Here's how the part is built. I have some questions about the finished solid (model axes, mm). Face numbers are marked on the shaded views. Coordinates: 2 decimals unless noted, no trailing zeros. Write each loop counter-clockwise with the first axis right and the second up, starting at its lowest first coordinate (ties: lowest second). Pieces come first, ordered by that corner, then holes.
Item 1: I'm going to push flat-ended pins straight in: pin 1 Ø5.5 at (x, y) = (-148.18, -60) entering from +Z; pin 2 Ø3 at (y, z) = (-53, -3) entering from +X; pin 3 Ø0.9 at (x, z) = (135.5, 10.5) entering from +Y; pin 4 Ø0.5 at (x, z) = (94.5, 9) entering from -Y. Where does each tip first touch, or does it pass through?
Item 2: We'd pull the mould along Z, two halves only. Please class the marked faces 1 and 2: +Z half, -Z half, draft (parallel to the pull), parting line (faces both ways), or undercut.
Item 3: If we section it at A-A (z = -5.5): Please give me the cut outline in (x, y).
Item 4: If we section it at B-B (x = -12.5): Please give me the cut outline in (y, z), then the cut area to 3 significant figures.
Item 5: If I drill on line 1 (Z direction, x = 17, y = 0); line 2 (Y direction, x = 98, z = 5.5), over which ranges is the centre line in solid material (lowest first)?
from build123d import *

# Parameters (mm, degrees)
SKETCH3_R               = 11
SKETCH3_R_2             = 10.2
CUT_EXTRUDE1_REACH      = 194.875
SKETCH4_R               = 3.5
SKETCH5_R               = 3.3
CUT_EXTRUDE2_DEPTH      = 193.875317702
CUT_EXTRUDE3_DEPTH      = 193.875317702
CUT_EXTRUDE3_DEPTH_BACK = 193.875317702


with BuildPart() as part:
    # Sweep2: sweep along a path in Sketch1
    with BuildLine(Plane.XY) as sweep2_path:
        Line((136.815388441, 0), (93.815388441, 0))
        Line((93.815388441, 0), (-93.815388441, 0))
        ThreePointArc((-93.815388441, 0), (-122.029080551, -9.16718427), (-139.466101223, -33.16718427))
        Line((-139.466101223, -33.16718427), (-148.184611559, -60))
        Line((-148.184611559, -60), (-157.932202446, -90))
    # Sketch3 → Sweep2 (sweep)
    with BuildSketch(Plane(origin=(93.815388441, 0, 0), x_dir=(0, 0, -1), z_dir=(1, 0, 0))):
        Circle(SKETCH3_R)
        Circle(SKETCH3_R_2, mode=Mode.SUBTRACT)
    sweep(path=sweep2_path.line)

    # Sketch4 → Cut-Extrude1 (cut, up to next)
    with BuildSketch(Plane.XY, mode=Mode.PRIVATE) as cut_extrude1_sk1:
        with Locations(Location((-148.184611559, -60, 0), (0, 0, 162))):
            Circle(SKETCH4_R)
    cut_extrude1_tool1 = extrude(cut_extrude1_sk1.sketch, amount=CUT_EXTRUDE1_REACH, mode=Mode.PRIVATE) & part.part
    # Sketch4 → Cut-Extrude1 (cut, up to next)
    with BuildSketch(Plane.XY, mode=Mode.PRIVATE) as cut_extrude1_sk2:
        with BuildLine():
            Line((91.815388441, -5.5), (95.815388441, -5.5))
            ThreePointArc((95.815388441, -5.5), (97.229602003, -4.914213562), (97.815388441, -3.5))
            Line((97.815388441, -3.5), (97.815388441, 3.5))
            ThreePointArc((97.815388441, 3.5), (97.229602003, 4.914213562), (95.815388441, 5.5))
            Line((95.815388441, 5.5), (91.815388441, 5.5))
            ThreePointArc((91.815388441, 5.5), (90.401174879, 4.914213562), (89.815388441, 3.5))
            Line((89.815388441, 3.5), (89.815388441, -3.5))
            ThreePointArc((89.815388441, -3.5), (90.401174879, -4.914213562), (91.815388441, -5.5))
        make_face()
    cut_extrude1_tool2 = extrude(cut_extrude1_sk2.sketch, amount=CUT_EXTRUDE1_REACH, mode=Mode.PRIVATE) & part.part
    add(cut_extrude1_tool1.solids().sort_by_distance((-148.184612, -60, 0))[0], mode=Mode.SUBTRACT)
    add(cut_extrude1_tool2.solids().sort_by_distance((93.815388, 0, 0))[0], mode=Mode.SUBTRACT)

    # Sketch5 → Cut-Extrude2 (cut, through all)
    with BuildSketch(Plane.XY):
        with Locations(Location((-148.184611559, -60, 0), (0, 0, 342))):
            Circle(SKETCH5_R)
    extrude(amount=-CUT_EXTRUDE2_DEPTH, mode=Mode.SUBTRACT)

    # Sketch6 → Cut-Extrude3 (cut, two sides: drawn at the far end of the back side and taken through both)
    with BuildSketch(Plane.XY.offset(-CUT_EXTRUDE3_DEPTH_BACK)):
        with BuildLine():
            Line((136.889174497, 2.554733627), (136.815388441, -2.554733627))
            Line((136.815388441, -2.554733627), (133.615388441, -2.554733627))
            ThreePointArc((133.615388441, -2.554733627), (132.201174879, -1.968947189), (131.615388441, -0.554733627))
            Line((131.615388441, -0.554733627), (131.615388441, 0.554733627))
            ThreePointArc((131.615388441, 0.554733627), (132.201174879, 1.968947189), (133.615388441, 2.554733627))
            Line((133.615388441, 2.554733627), (136.889174497, 2.554733627))
        make_face()
    extrude(amount=CUT_EXTRUDE3_DEPTH + CUT_EXTRUDE3_DEPTH_BACK, mode=Mode.SUBTRACT)


solid = part.part
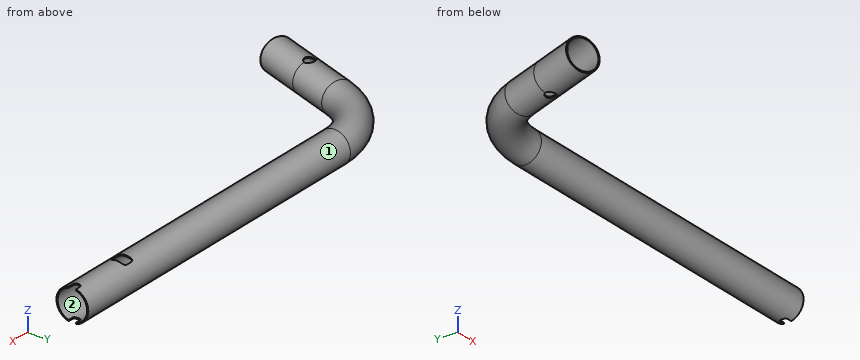
Answer list:
1. pin 1: passes through
1. pin 2: stops at x = -134.17
1. pin 3: stops at y = 4.47
1. pin 4: stops at y = -6.67
2. face 1: parting line
2. face 2: undercut
3. outline: (-166.99, -87.06) - (-166.1, -87.35) - (-147.64, -30.51) arc R56.59 cw to (-93.82, 8.59) - (136.82, 8.59) - (136.82, 9.53) - (-93.82, 9.53) arc R57.53 ccw to (-148.53, -30.22) - close; (-149.76, -92.65) - (-148.87, -92.94) - (-130.41, -36.11) arc R38.47 cw to (-93.82, -9.53) - (136.82, -9.53) - (136.82, -8.59) - (-93.82, -8.59) arc R39.41 ccw to (-131.3, -35.82) - close
4. outline: circle Ø22 at (0, 0); hole circle Ø20.4 at (0, 0)
4. area: 53.3 mm2
5. line 1: z = -11 to -10.2, 10.2 to 11
5. line 2: y = -9.53 to -8.59, 8.59 to 9.53
